Geometry check sheet. Reference: the model listing, model coordinates, mm. Give positions to 0.01 mm unless a question says otherwise; leave off trailing zeros. Loops run counter-clockwise (first coordinate to the right, second up) from the corner with the lowest first, then second, coordinate; pieces in that order, holes last. Notation, with made-up numbers: (-5, -19.75) -> (35, -19.75) arc R25 ccw to (35, -1.75) -> close; hole circle Ø6 at (-19.5, 8). An arc over 180 degrees is marked (long way). One line per item, written item: value. Start each with the question number.
(1) Sectioned sample at B-B, the plane z = 80. Record the cut outline in (x, y) (3 decimals), then the cut area to 3 significant figures.
(2) Gauge pin test, flat ends, axial feed: pin 1 Ø1.8 at (y, z) = (-1.5, 181.5) entering from +X; pin 2 Ø0.7 at (x, y) = (74.5, -1.5) entering from -Z; pin 3 Ø1 at (x, z) = (49, 56.5) entering from +Y; pin 4 Ø1.2 at (x, y) = (-69.5, -1) entering from +Z. Record the tip position at first contact, or that the pin passes through.
(3) Scan lines: line 1 along X through (y, z) = (-1.8, 16); line 2 along Z through (x, y) = (24.5, -1.05); line 3 along X through (y, z) = (-2.15, -3). Record each from-to range of solid material in increasing order. Write a range as from..to.
(4) Sectioned sample at A-A, the plane z = -6.5. Record the cut outline in (x, y) (3 decimals).
from build123d import *

# Parameters (mm, degrees)
F1_DEPTH = 3.175


# Not quite as in the source:
# - ends of sketch curves that miss each other by under 0.0002 mm in the source are joined


with BuildPart() as f1:
    # F0 (on Front) → F1 (new body)
    with BuildSketch(Plane.XZ):
        Polygon((-0.0247448797, 196.3262024198), (-79.3997448797, 196.3262024198), (-79.3997448797, 193.1512024198), (-76.2247448797, 193.1512024198), (-76.2247448797, 185.2391024198), (-73.8117448797, 185.2391024198), (-73.8117448797, 186.8520024198), (-70.6367448797, 186.8520024198), (-70.6367448797, 185.2391024198), (-68.2745449228, 185.2899024198), (-68.2745449228, 182.1149024198), (-70.6367449228, 182.1149024198), (-70.6367449228, 180.5020024198), (-73.8117449228, 180.5020024198), (-73.8117449228, 182.1149024198), (-76.2247448797, 182.1149024198), (-76.2247448797, 174.1012024198), (-79.3997448797, 174.1012024198), (-79.3997448797, 170.9262024198), (-76.2247448797, 170.9262024198), (-76.2247448797, 113.7762024198), (-79.3997448797, 113.7762024198), (-79.3997421861, 110.6520024198), (-76.2247421861, 110.6520024198), (-76.2247421861, 102.7399024198), (-73.8117421861, 102.7399024198), (-73.8117421861, 104.3528024198), (-70.6367421861, 104.3528024198), (-70.6367421861, 102.7399024198), (-68.2745421861, 102.7907024198), (-68.2745421861, 99.6157024198), (-70.6367421861, 99.6157024198), (-70.6367421861, 98.0028024198), (-73.8117421861, 98.0028024198), (-73.8117421861, 99.6157024198), (-76.2247421861, 99.6157024198), (-76.2247421861, 91.5512024198), (-79.3997421861, 91.5512024198), (-79.3997421861, 88.3762024198), (-76.2247449228, 88.3762024198), (-76.2247449228, 31.2262024198), (-79.3997448797, 31.2262024198), (-79.3997421861, 28.0512024198), (-76.2247421861, 28.0512024198), (-76.2247421861, 20.1391024198), (-73.8117421861, 20.1391024198), (-73.8117421861, 21.7520024198), (-70.6367421861, 21.7520024198), (-70.6367421861, 20.1391024198), (-68.2745421861, 20.1899024198), (-68.2745421861, 17.0149024198), (-70.6367421861, 17.0149024198), (-70.6367421861, 15.4020024198), (-73.8117421861, 15.4020024198), (-73.8117421861, 17.0149024198), (-76.2247421861, 17.0149024198), (-76.2247421861, 9.0012024198), (-79.3997421861, 9.0012024198), (-79.3997421861, 5.8262024198), (-76.2247421861, 5.8262024198), (-76.2247421861, -34.6613975802), (0, -34.6613975802), align=None)
        Polygon((79.3502532985, 196.3432087423), (-0.0247448797, 196.3262024198), (0, -34.6613975802), (76.2247404365, -34.6450662095), (76.2160658516, 5.8425328612), (79.3910657787, 5.8432131141), (79.3903855258, 9.0182130412), (76.2153855987, 9.0175327883), (76.2136686404, 17.0312326044), (73.8006686958, 17.0307156122), (73.8010142642, 15.4178156492), (70.6260143371, 15.4171353963), (70.6256687686, 17.0300353593), (68.2634688228, 17.0295292511), (68.2627885699, 20.2045291783), (70.6249993998, 20.1542352876), (70.6246538313, 21.7671352506), (73.7996537584, 21.7678155035), (73.7999993269, 20.1549155405), (76.2129992715, 20.1554325327), (76.2113040813, 28.0675323511), (79.3863040084, 28.068212604), (79.3856264492, 31.2432125317), (76.2106265651, 31.2425322788), (76.198382013, 88.3925309671), (79.3733792034, 88.3932112194), (79.3726989505, 91.5682111465), (76.1976990233, 91.5675308936), (76.195971181, 99.6320307085), (73.7829712364, 99.6315137163), (73.7833168048, 98.0186137533), (70.6083168777, 98.0179335004), (70.6079713092, 99.6308334634), (68.2457713634, 99.6303273553), (68.2450911105, 102.8053272824), (70.6073019404, 102.7550333917), (70.6069563719, 104.3679333547), (73.781956299, 104.3686136076), (73.7823018675, 102.7557136446), (76.1953018121, 102.7562306368), (76.1936066219, 110.6683304552), (79.368606549, 110.6690107081), (79.3679371802, 113.7932106364), (76.1929399467, 113.7925303841), (76.1806953945, 170.9425290724), (79.3556953216, 170.9432093253), (79.3550150687, 174.1182092524), (76.1800151416, 174.1175289995), (76.1782981833, 182.1312288156), (73.7652982818, 182.1307118234), (73.7656438503, 180.5178118604), (70.5906439231, 180.5171316075), (70.5902983547, 182.1300315705), (68.2280984089, 182.1295254623), (68.227418156, 185.3045253894), (70.5896289427, 185.2542314987), (70.5892833742, 186.8671314617), (73.7642833014, 186.8678117146), (73.7646288698, 185.2549117516), (76.1776288145, 185.2554287439), (76.1759336242, 193.1675285623), (79.3509335514, 193.1682088151), align=None)
    extrude(amount=F1_DEPTH)


solid = f1.part
Calculated:
1. outline: (-76.225, -3.175) -> (76.2, -3.175) -> (76.2, 0) -> (-76.225, 0) -> close
1. area: 484 mm2
2. pin 1: stops at x = 76.18
2. pin 2: stops at z = -34.65
2. pin 3: stops at y = 0
2. pin 4: stops at z = 196.33
3. line 1: x = -76.22..-73.81, -70.64..70.63, 73.8..76.21
3. line 2: z = -34.66..196.33
3. line 3: x = -76.22..76.22
4. outline: (-76.225, -3.175) -> (76.219, -3.175) -> (76.219, 0) -> (-76.225, 0) -> close
